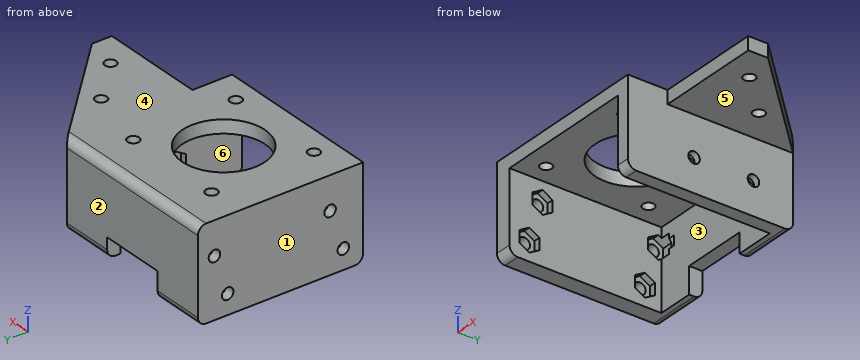
from build123d import *

# Parameters (mm, degrees)
BOSS_EXTRUDE1_DEPTH      = 4
SKETCH2_R                = 12.5
SKETCH2_R_2              = 1.75
CUT_EXTRUDE1_DEPTH       = 5
SKETCH9_R                = 1.75
CUT_EXTRUDE2_DEPTH       = 4
BOSS_EXTRUDE8_DEPTH      = 24
SKETCH18_R               = 1.75
CUT_EXTRUDE7_DEPTH       = 4
SKETCH19_R               = 1.75
CUT_EXTRUDE8_DEPTH       = 10
CUT_EXTRUDE9_DEPTH       = 50
FILLET1_R                = 2.5
CUT_EXTRUDE11_DEPTH      = 3
CUT_EXTRUDE11_DEPTH_BACK = 2
CUT_EXTRUDE12_DEPTH      = 2
CUT_EXTRUDE13_DEPTH      = 2
FILLET2_R                = 2.5


with BuildPart() as part:
    # Sketch1 → Boss-Extrude1 (new body)
    with BuildSketch(Plane.XY):
        Polygon((57.5, 18), (25.5, 50), (-26.5, 50), (-26.5, 0), (25.5, 0), (25.5, 12), (57.5, 12), align=None)
    extrude(amount=BOSS_EXTRUDE1_DEPTH)

    # Sketch2 → Cut-Extrude1 (cut, through all)
    with BuildSketch(Plane.XY.offset(4)):
        with Locations((0, 22)):
            Circle(SKETCH2_R)
        with Locations((15.5, 6.5)):
            Circle(SKETCH2_R_2)
        with Locations((15.5, 37.5)):
            Circle(SKETCH2_R_2)
        with Locations((-15.5, 37.5)):
            Circle(SKETCH2_R_2)
        with Locations((-15.5, 6.5)):
            Circle(SKETCH2_R_2)
    extrude(amount=-CUT_EXTRUDE1_DEPTH, mode=Mode.SUBTRACT)

    # Sketch9 → Cut-Extrude2 (cut)
    with BuildSketch(Plane(origin=(0, 0, 0), x_dir=(-1, 0, 0), z_dir=(0, 0, -1))):
        with Locations((-47.5, 20)):
            Circle(SKETCH9_R)
        with Locations((-35.5, 32)):
            Circle(SKETCH9_R)
    extrude(amount=-CUT_EXTRUDE2_DEPTH, mode=Mode.SUBTRACT)

    # Sketch17 → Boss-Extrude8 (add)
    with BuildSketch(Plane(origin=(0, 0, 0), x_dir=(-1, 0, 0), z_dir=(0, 0, -1))):
        Polygon((-25.5, 0), (-25.5, 50), (26.5, 50), (26.5, 0), (21.5, 0), (21.5, 46), (-21.5, 46), (-21.5, 0), align=None)
    extrude(amount=BOSS_EXTRUDE8_DEPTH)

    # Sketch18 → Cut-Extrude7 (cut)
    with BuildSketch(Plane(origin=(25.5, 0, 0), x_dir=(0, 0, -1), z_dir=(1, 0, 0))):
        with Locations((12, 38)):
            Circle(SKETCH18_R)
        with Locations((12, 20)):
            Circle(SKETCH18_R)
    extrude(amount=-CUT_EXTRUDE7_DEPTH, mode=Mode.SUBTRACT)

    # Sketch19 → Cut-Extrude8 (cut)
    with BuildSketch(Plane.ZY.offset(26.5)):
        with Locations((-18, 6)):
            Circle(SKETCH19_R)
        with Locations((-18, 41)):
            Circle(SKETCH19_R)
        with Locations((-6, 10)):
            Circle(SKETCH19_R)
        with Locations((-6, 45)):
            Circle(SKETCH19_R)
    extrude(amount=-CUT_EXTRUDE8_DEPTH, mode=Mode.SUBTRACT)

    # Sketch20 → Cut-Extrude9 (cut)
    with BuildSketch(Plane(origin=(0, 50, 0), x_dir=(1, 0, 0), z_dir=(0, 1, 0))):
        Polygon((25.5, 24), (-10.5, 24), (-10.5, 16), (9.5, 16), (9.5, 22), (25.5, 22), align=None)
    extrude(amount=-CUT_EXTRUDE9_DEPTH, mode=Mode.SUBTRACT)

    # Fillet1
    fillet1_edges = [part.edges().sort_by_distance(p)[0] for p in [
        (23.5, 0, -22),
        (17.5, 50, -22),
        (-24, 0, -24),
        (-18.5, 50, -24),
    ]]
    fillet(fillet1_edges, radius=FILLET1_R)

    # Sketch22 → Cut-Extrude11 (cut, two sides)
    with BuildSketch(Plane(origin=(-21.5, 0, 0), x_dir=(0, 0, -1), z_dir=(1, 0, 0))) as cut_extrude11_sk:
        Polygon((7.75, 41.968911087), (9.5, 45), (7.75, 48.031088913), (4.25, 48.031088913), (2.5, 45), (4.25, 41.968911087), align=None)
    extrude(amount=CUT_EXTRUDE11_DEPTH, mode=Mode.SUBTRACT)
    extrude(cut_extrude11_sk.sketch, amount=-CUT_EXTRUDE11_DEPTH_BACK, mode=Mode.SUBTRACT)

    # Sketch23 → Cut-Extrude12 (cut)
    with BuildSketch(Plane(origin=(-21.5, 0, 0), x_dir=(0, 0, -1), z_dir=(1, 0, 0))):
        Polygon((19.75, 37.968911087), (21.5, 41), (19.75, 44.031088913), (16.25, 44.031088913), (14.5, 41), (16.25, 37.968911087), align=None)
        Polygon((7.75, 6.968911087), (9.5, 10), (7.75, 13.031088913), (4.25, 13.031088913), (2.5, 10), (4.25, 6.968911087), align=None)
        Polygon((16.25, 2.968911087), (19.75, 2.968911087), (21.5, 6), (19.75, 9.031088913), (16.25, 9.031088913), (14.5, 6), align=None)
    extrude(amount=-CUT_EXTRUDE12_DEPTH, mode=Mode.SUBTRACT)

    # Sketch24 → Cut-Extrude13 (cut)
    with BuildSketch(Plane.ZY.offset(-21.5)):
        Polygon((-10.240287428, 41.047911581), (-13.759712572, 41.047911581), (-15.519425144, 38), (-13.759712572, 34.952088419), (-10.240287428, 34.952088419), (-8.480574856, 38), align=None)
        Polygon((-10.25, 23.031088913), (-13.75, 23.031088913), (-15.5, 20), (-13.75, 16.968911087), (-10.25, 16.968911087), (-8.5, 20), align=None)
    extrude(amount=-CUT_EXTRUDE13_DEPTH, mode=Mode.SUBTRACT)

    # Fillet2
    fillet2_edges = [part.edges().sort_by_distance(p)[0] for p in [
        (-0.5, 50, 4),
    ]]
    fillet(fillet2_edges, radius=FILLET2_R)


solid = part.part
Can you work these out from the model? Positions are in its coordinate system, mm. Face numbers are marked on the shaded views. A direction names the side the tool comes from. Coordinates: 2 decimals unless noted, no trailing zeros. Write each loop counter-clockwise with the first axis right and the second up, starting at its lowest first coordinate (ties: lowest second). Pieces come first, ordered by that corner, then holes. Notation, with made-up numbers: (-16, 41.25) -> (42, 41.25) arc R20 cw to (42, 50.25) -> close; hole circle Ø4 at (24, 19). An arc over 180 degrees is marked (long way). Write item = value, one per line.
(1) Imagine slicing it at D-D (x = 0). Please give me the cut outline in (y, z), and give its area (3 significant figures).
Verdict:
outline = (0, 0) -> (9.5, 0) -> (9.5, 4) -> (0, 4) -> close; (34.5, 0) -> (46, 0) -> (46, -16) -> (50, -16) -> (50, 1.5) arc R2.5 ccw to (47.5, 4) -> (34.5, 4) -> close
area = 163 mm^2
(2) On a 3-axis mill with a long thin cutter (end or side, diameter ignored), from which of +Z, -Z, +X, -X, +Y, -Y can I reach the whole of each face in a straight line? I mean the marked faces 4, 5 and 6. Say none if no direction works.
Verdict:
face_4 = +Z, +X, -X, +Y, -Y
face_5 = -Z, +X, +Y, -Y
face_6 = -Z, -Y
(3) For pin 1 (3 mm diameter, centred on y = 7.5, z = -19, fed in from +X); pin 2 (2 mm diameter, centred on x = -3, y = 47, fed in from -Z); pin 3 (5 mm diameter, centred on x = 0.5, y = 32.5, fed in from +Z); pin 4 (4.5 mm diameter, centred on x = 47.5, y = 20, fed in from -Z), each with a flat end and sliding along its axis, tell me the tip position at first contact or that it passes through.
Verdict:
pin_1 = 25.5
pin_2 = -16
pin_3 = 4
pin_4 = 0
(4) Imagine slicing it at A-A (x = 15.5). Please give me the cut outline in (y, z), and give its area (3 significant figures).
Verdict:
outline = (0, 0) -> (4.75, 0) -> (4.75, 4) -> (0, 4) -> close; (8.25, 0) -> (35.75, 0) -> (35.75, 4) -> (8.25, 4) -> close; (39.25, 0) -> (46, 0) -> (46, -22) -> (47.5, -22) arc R2.5 ccw to (50, -19.5) -> (50, 1.5) arc R2.5 ccw to (47.5, 4) -> (39.25, 4) -> close
area = 257 mm^2
(5) Imagine slicing it at B-B (y = 32). Please give me the cut outline in (x, z).
Verdict:
outline = (-26.5, -24) -> (-21.5, -24) -> (-21.5, 0) -> (-7.5, 0) -> (-7.5, 4) -> (-26.5, 4) -> close; (7.5, 0) -> (21.5, 0) -> (21.5, -22) -> (25.5, -22) -> (25.5, 0) -> (33.75, 0) -> (33.75, 4) -> (7.5, 4) -> close; (37.25, 0) -> (43.5, 0) -> (43.5, 4) -> (37.25, 4) -> close
(6) Thinking about a two-plate mould opening in X: for the marked faces 1, 2 and 3, which applies, +X half, -X half, draft (parallel to the pull), parting line (faces both ways), or undercut?
Verdict:
face_1 = -X half
face_2 = draft
face_3 = undercut
(7) Imagine slicing it at C-C (z = -12). Please give me the cut outline in (x, y).
Verdict:
outline = (-26.5, 0) -> (-21.5, 0) -> (-21.5, 46) -> (21.5, 46) -> (21.5, 41.05) -> (23.5, 41.05) -> (23.5, 39.75) -> (25.5, 39.75) -> (25.5, 50) -> (-26.5, 50) -> close; (21.5, 0) -> (25.5, 0) -> (25.5, 18.25) -> (23.5, 18.25) -> (23.5, 16.97) -> (21.5, 16.97) -> close; (21.5, 23.03) -> (23.5, 23.03) -> (23.5, 21.75) -> (25.5, 21.75) -> (25.5, 36.25) -> (23.5, 36.25) -> (23.5, 34.95) -> (21.5, 34.95) -> close
(8) If I drill on probe 1 along Y at (x, z) = (-15.5, 1.4); probe 2 along Y at (x, z) = (-25.3, -18); probe 3 along X at (y, z) = (31.5, -4.75), over which ranges is the centre line in solid material (lowest first)?
Verdict:
probe_1 = 0 to 4.75, 8.25 to 35.75, 39.25 to 50
probe_2 = 0 to 4.25, 7.75 to 39.25, 42.75 to 50
probe_3 = -26.5 to -21.5, 21.5 to 25.5
